Verification items for this drawing (mm, ordinates from the low corner). A direction names the side the tool comes from. Coordinates: 2 decimals unless noted, no trailing zeros. Order: outer loops, then holes, each group sorted by start corner. A loop starts at its lowest first (then second) coordinate and runs counter-clockwise, first axis right, second up.
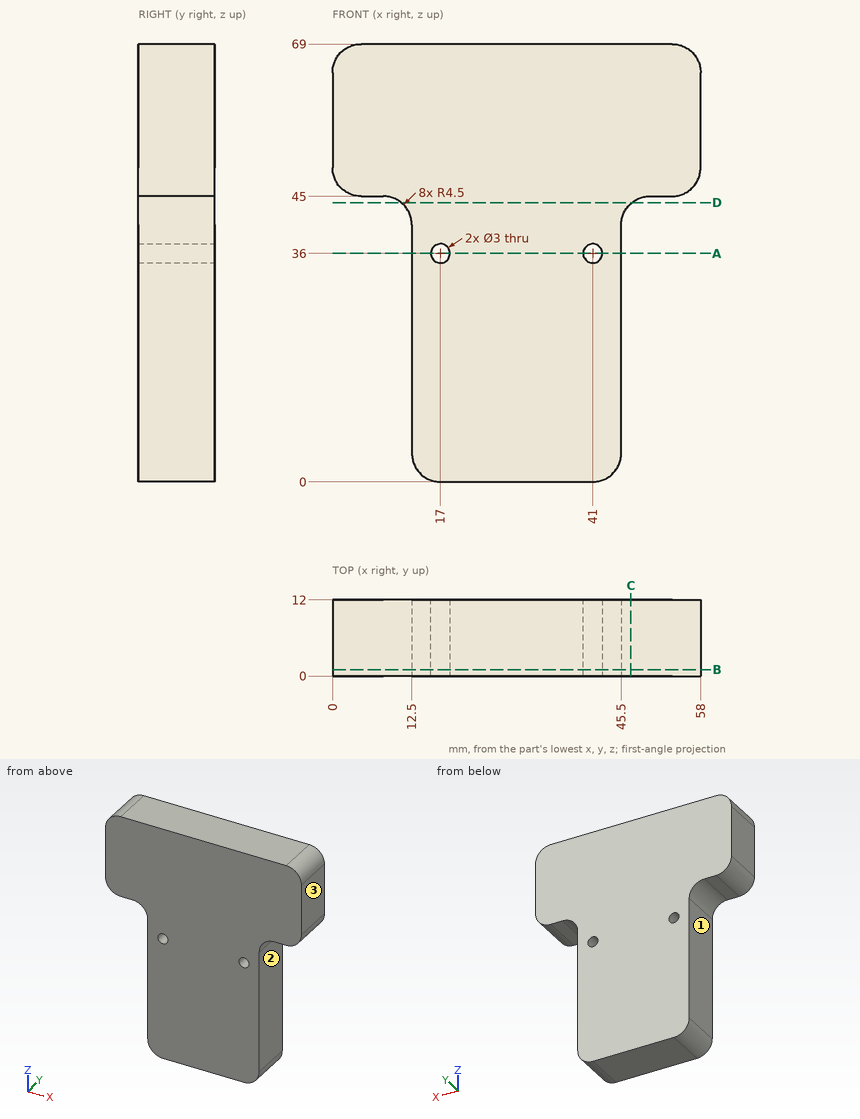
(1) Tool access check on the marked faces 1, 2 and 3. Record the directions out of +Z, -Z, +X, -X, +Y, -Y that give a thin tool (end or side, any length) a straight path to the whole face; none if there is none.
Filled in:
face 1: -Z, -X, +Y, -Y
face 2: -Z, +X, +Y, -Y
face 3: +Z, -Z, +X, +Y, -Y
(2) Cross-section at C-C (x = 47). Enter the section's corners in (y, z).
Filled in:
outline: (0, 43.85) - (12, 43.85) - (12, 69) - (0, 69) - close
(3) Cross-section at A-A (z = 36). Enter the section's corners in (x, y), and give its area (3 significant figures).
Filled in:
outline: (12.5, 0) - (15.5, 0) - (15.5, 12) - (12.5, 12) - close; (18.5, 0) - (39.5, 0) - (39.5, 12) - (18.5, 12) - close; (42.5, 0) - (45.5, 0) - (45.5, 12) - (42.5, 12) - close
area: 324 mm2
(4) Cross-section at B-B (y = 1). Enter the section's corners in (x, z), and give its area (3 significant figures).
Filled in:
outline: (0, 49.5) arc R4.5 ccw to (4.5, 45) - (8, 45) arc R4.5 cw to (12.5, 40.5) - (12.5, 4.5) arc R4.5 ccw to (17, 0) - (41, 0) arc R4.5 ccw to (45.5, 4.5) - (45.5, 40.5) arc R4.5 cw to (50, 45) - (53.5, 45) arc R4.5 ccw to (58, 49.5) - (58, 64.5) arc R4.5 ccw to (53.5, 69) - (4.5, 69) arc R4.5 ccw to (0, 64.5) - close; hole circle Ø3 at (17, 36); hole circle Ø3 at (41, 36)
area: 2,850 mm2
(5) Go/stop test with flat-tipped pins: P1, Ø3, axis at y = 9, z = 23.5, coming from the -X side; P2, Ø4, axis at x = 5.5, y = 6, coming from the -Z side. Record where each tip stops, or that it passes through.
Filled in:
P1: stops at x = 12.5
P2: stops at z = 45
(6) Cross-section at D-D (z = 44). Enter the section's corners in (x, y).
Filled in:
outline: (10.83, 0) - (47.17, 0) - (47.17, 12) - (10.83, 12) - close
(7) Thickness scan on probe 1 along X at (y, z) = (1.5, 26); probe 2 along Z at (x, y) = (7, 3.75); probe 3 along X at (y, z) = (9.25, 45.5). Record the ranges inside material, lowest first.
Filled in:
probe 1: x = 12.5 to 45.5
probe 2: z = 45 to 69
probe 3: x = 2.44 to 55.56
